For this review, take the finished solid that the model builds, in its own axes (mm). Face numbers are marked on the shaded views. A direction names the side the tool comes from. Give positions to 0.01 mm unless a question says otherwise; leave off trailing zeros. Order: outer loops, then holes, each group sorted by start corner. A loop starts at its lowest first (then second) coordinate and runs counter-clockwise, first axis right, second up. Notation, with made-up numbers: M 44.25,17 L 66.25,17 A19 ccw 66.25,23 Z; hole C 30.25,-6.75 d8. An arc over 180 degrees is marked long. Answer as CSV lines item,"result". Start each with the question number.
1. Mouldability with a two-part tool opening along Y and no side actions: class the marked faces 1, 2, 3 and 4 as pulls with the +Y half, pulls with the -Y half, needs draft (parallel to the pull), parting line crosses it, or undercut.
2. We need section D-D, the plane y = 4. Give the boundary of the cut face in (x, z) (1 decimal), and give its area (3 significant figures).
3. We need section C-C, the plane y = 6. Give the boundary of the cut face in (x, z) (1 decimal), and give its area (3 significant figures).
4. Machinability: for the marked faces 5 and 6, which of the approach directions +Z, -Z, +X, -X, +Y, -Y give a long, thin tool a straight path to every point of the face, cutting with its end or side? Answer none if there is none.
5. Clearance check with flat-ended pins moving along their axes: P1, Ø1.9, axis at x = 0, z = 0, coming from the -Y side; P2, Ø1, axis at x = 1.5, y = 5, coming from the -Z side; P3, Ø1.5, axis at y = 3.5, z = -2, coming from the -X side. State where each tip first meets the part, or that it passes through.
6. For line 1 along X through (y, z) = (0, 0.1); line 2 along Z through (x, y) = (0, 2.25); line 3 along Z through (x, y) = (0.9, 5), list the stretches that pass through material, from the lowest coordinate up.
Autodesk Inventor part; units mm, degrees
ref_plane "YZ Plane" through (0, 0, 0) normal (1, 0, 0) x (0, 1, 0)
ref_plane "XZ Plane" through (0, 0, 0) normal (0, 1, 0) x (-1, 0, 0)
ref_plane "XY Plane" through (0, 0, 0) normal (0, 0, 1) x (1, 0, 0)
sketch "Sketch1" plane through (0, 0, 0) normal (0, 0, 1) x (1, 0, 0)
  line L0 (1.5875, 0) -> (1.5875, 8.89)
  line L1 (1.5875, 8.89) -> (2.4832, 3.81)
  line L2 (1.5875, 8.89) -> (6.7459, 8.89) construction
  line L3 (2.4832, 3.81) -> (2.085, 3.81)
  line L4 (2.085, 3.81) -> (2.4832, 1.5517)
  line L5 (2.4832, 1.5517) -> (1.8611, 1.5517)
  line L6 (1.8611, 1.5517) -> (1.8611, 0)
  line L7 (1.8611, 0) -> (1.5875, 0)
  line L8 (0, -4.826) -> (0, 11.176)
  line L9 (1.5875, 0) -> (1.8611, 0)
  line L10 (1.8611, 0) -> (1.8611, -2.54) construction
  line L11 (1.8611, -2.54) -> (1.5875, -2.54) construction
  line L12 (1.5875, -2.54) -> (1.5875, 0) construction
  line L13 (1.5875, 0) -> (1.0583, -2.54)
  line L14 (1.0583, -2.54) -> (1.5875, -2.54) construction
  line L15 (1.8611, 0) -> (1.3319, -2.54)
  line L16 (1.0583, -2.54) -> (1.3319, -2.54)
  point P0 (0, 0)
  point P1 (2.1722, 1.5517)
  dimension "d1" = 1.5875
  dimension "d3" = 0
  dimension "d4" = 80
  dimension "d5" = 0.3982
  dimension "d6" = 2.2583
  dimension "d7" = 1.5517
  dimension "d8" = 1.8611
  dimension "d10" = 8.89
  dimension "d11" = 2.54
  dimension "d12" = 0.2736
  dimension "d17" = 0.2736
  dimension "d18" = 1.0583
revolve "Revolution2" add sketch "Sketch1" angle 360 about axis through (0, -10, 0) along (0, 1, 0)
properties part number "eigthinch"
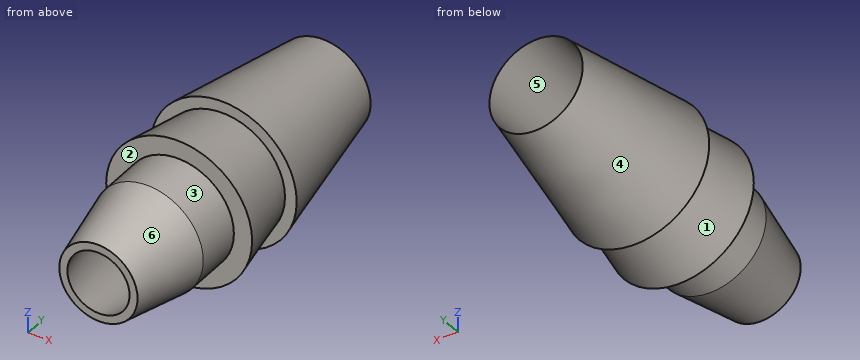
Result set:
1,face 1,"undercut"
1,face 2,"pulls with the -Y half"
1,face 3,"needs draft"
1,face 4,"pulls with the +Y half"
2,outline,"C 0,0 d4.9; hole C 0,0 d3.2"
2,area,"10.9 mm2"
3,outline,"C 0,0 d4.2; hole C 0,0 d3.2"
3,area,"5.90 mm2"
4,face 5,"+Y"
4,face 6,"-Y"
5,P1,"through"
5,P2,"z = -2.06"
5,P3,"x = -2.11"
6,line 1,"-1.86 to -1.58, 1.58 to 1.86"
6,line 2,"-2.36 to -1.59, 1.59 to 2.36"
6,line 3,"-2.09 to -1.31, 1.31 to 2.09"
